Read the model definition and answer for the solid it produces. Units are mm, in the model's axes. Face numbers are marked on the shaded views. A direction names the side the tool comes from. Give positions to 0.01 mm unless a question says otherwise; leave off trailing zeros. Loops run counter-clockwise (first coordinate to the right, second up) from the corner with the lowest first, then second, coordinate; pieces in that order, holes last. Notation, with made-up numbers: (-6.5, 78) - (48.5, 78) arc R26 ccw to (48.5, 116) - close; hole circle Ø9 at (21, 72.5). An arc over 180 degrees is marked (long way). Put each result on its own line as item: value. Start each with the question number.
1. For a pull along X with two mould halves and no side action, classify the marked faces 1, 2 and 3 as released by +X, released by -X, zero draft, split by the parting line, or undercut.
2. Consider L1, parallel to Z at x = -20, y = 6; L2, parallel to Y at x = -5, z = -15; L3, parallel to Y at x = 2, z = 20. Determine where each line is inside the solid, lowest interval first. Write a range as from..to.
3. A cutting plane is placed at C-C, the plane z = 2. Determine the outline of the cut face in (x, y).
4. A cutting plane is placed at B-B, the plane x = -16.5. Determine the outline of the cut face in (y, z).
5. A cutting plane is placed at D-D, the plane x = -58. Determine the outline of the cut face in (y, z), plus the area to 3 significant figures.
6. For the marked faces 4, 5 and 6, determine the directions among +Z, -Z, +X, -X, +Y, -Y from which every point of the face is accessible in a straight line to the end or side of a thin tool.
7. A cutting plane is placed at A-A, the plane y = 9. Determine the outline of the cut face in (x, z).
8. Given pin 1 Ø24 at (y, z) = (40.5, -5.5) entering from -X; pin 2 Ø1.3 at (x, z) = (29.5, 28) entering from +Y; pin 3 Ø11.5 at (x, z) = (-11.5, 31) entering from +Y, each flat-ended and moving along its own axis, determine where each tip first touches the part or whether it passes through.
```python
from build123d import *

# Parameters (mm, degrees)
SKETCH_W     = 60
SKETCH_H     = 85
PAD_DEPTH    = 1.2
SKETCH002_W  = 60
SKETCH002_H  = 1.2
PAD001_DEPTH = 80
SKETCH003_W  = 60
SKETCH003_H  = 1.2
PAD002_DEPTH = 60
SKETCH004_W  = 60
SKETCH004_H  = 1.2
PAD003_DEPTH = 35
SKETCH006_W  = 60
SKETCH006_H  = 2.4
PAD004_DEPTH = 4
SKETCH005_W  = 11.7
SKETCH005_H  = 2.4
PAD005_DEPTH = 18.6
SKETCH007_W  = 17
SKETCH007_H  = 0.8
PAD006_DEPTH = 36.6
SKETCH009_W  = 61.2
SKETCH009_H  = 1.2
PAD007_DEPTH = 35
SKETCH010_W  = 1.2
SKETCH010_H  = 60
PAD008_DEPTH = 78.8
SKETCH011_W  = 1.2
SKETCH011_H  = 22.6
PAD009_DEPTH = 32.6
FILLET_R     = 1
FILLET001_R  = 1
FILLET002_R  = 1
FILLET003_R  = 1
FILLET004_R  = 1
FILLET005_R  = 1
FILLET006_R  = 1
FILLET007_R  = 1
FILLET008_R  = 1
FILLET009_R  = 1
FILLET010_R  = 1
FILLET011_R  = 1
FILLET012_R  = 1
FILLET013_R  = 1
FILLET014_R  = 0.4
FILLET015_R  = 0.4
SKETCH012_W  = 16
SKETCH012_H  = 8
POCKET_DEPTH = 95.001


with BuildPart() as part:
    # Sketch → Pad (new body)
    with BuildSketch(Plane.XZ):
        Rectangle(SKETCH_W, SKETCH_H)
    extrude(amount=PAD_DEPTH)

    # Sketch002 (on Face5 of Pad) → Pad001 (join)
    with BuildSketch(Plane(origin=(0, 0, 0), x_dir=(1, 0, 0), z_dir=(0, 1, 0))):
        with Locations((0, 41.9)):
            Rectangle(SKETCH002_W, SKETCH002_H)
    extrude(amount=PAD001_DEPTH)

    # Sketch003 (on Face4 of Pad001) → Pad002 (join)
    with BuildSketch(Plane(origin=(0, 0, -41.3), x_dir=(-1, 0, 0), z_dir=(0, 0, 1))):
        with Locations((0, -79.4)):
            Rectangle(SKETCH003_W, SKETCH003_H)
    extrude(amount=PAD002_DEPTH)

    # Sketch004 (on Face2 of Pad002) → Pad003 (join)
    with BuildSketch(Plane(origin=(0, 0, 0), x_dir=(1, 0, 0), z_dir=(0, 1, 0))):
        with Locations((0, -41.9)):
            Rectangle(SKETCH004_W, SKETCH004_H)
    extrude(amount=PAD003_DEPTH)

    # Sketch006 (on Face7 of Pad003) → Pad004 (join)
    with BuildSketch(Plane(origin=(0, 0, 41.3), x_dir=(1, 0, 0), z_dir=(0, 0, -1))):
        with Locations((0, -33.8)):
            Rectangle(SKETCH006_W, SKETCH006_H)
    extrude(amount=PAD004_DEPTH)

    # Sketch005 (on Face11 of Pad004) → Pad005 (join)
    with BuildSketch(Plane(origin=(0, 0, 37.3), x_dir=(1, 0, 0), z_dir=(0, 0, -1))):
        with Locations((24.15, -33.8)):
            Rectangle(SKETCH005_W, SKETCH005_H)
        with Locations((-24.15, -33.8)):
            Rectangle(SKETCH005_W, SKETCH005_H)
    extrude(amount=PAD005_DEPTH)

    # Sketch007 (on Face12 of Pad005) → Pad006 (join)
    with BuildSketch(Plane(origin=(-18.3, 0, 0), x_dir=(0, 0, 1), z_dir=(1, 0, 0))):
        with Locations((28, -33.8)):
            Rectangle(SKETCH007_W, SKETCH007_H)
    extrude(amount=PAD006_DEPTH)

    # Sketch009 (on Face2 of Pad006) → Pad007 (join)
    with BuildSketch(Plane(origin=(-30, 0, 0), x_dir=(0, 0, -1), z_dir=(-1, 0, 0))):
        with Locations((11.9, -79.4)):
            Rectangle(SKETCH009_W, SKETCH009_H)
    extrude(amount=PAD007_DEPTH)

    # Sketch010 (on Face22 of Pad007) → Pad008 (join)
    with BuildSketch(Plane.XZ.offset(-78.8)):
        with Locations((29.4, -11.3)):
            Rectangle(SKETCH010_W, SKETCH010_H)
    extrude(amount=PAD008_DEPTH)

    # Sketch011 (on Face9 of Pad008) → Pad009 (join)
    with BuildSketch(Plane.XZ.offset(-32.6)):
        with Locations((29.4, 30)):
            Rectangle(SKETCH011_W, SKETCH011_H)
    extrude(amount=PAD009_DEPTH)

    # Fillet
    fillet_edges = [part.edges().sort_by_distance(p)[0] for p in [
        (0, 35, 42.5),
    ]]
    fillet(fillet_edges, radius=FILLET_R)

    # Fillet001
    fillet001_edges = [part.edges().sort_by_distance(p)[0] for p in [
        (0, -1.2, 42.5),
    ]]
    fillet(fillet001_edges, radius=FILLET001_R)

    # Fillet002
    fillet002_edges = [part.edges().sort_by_distance(p)[0] for p in [
        (-0.6, 0, 41.3),
    ]]
    fillet(fillet002_edges, radius=FILLET002_R)

    # Fillet003
    fillet003_edges = [part.edges().sort_by_distance(p)[0] for p in [
        (-0.6, 32.6, 41.3),
    ]]
    fillet(fillet003_edges, radius=FILLET003_R)

    # Fillet004
    fillet004_edges = [part.edges().sort_by_distance(p)[0] for p in [
        (-24.15, 32.6, 18.7),
    ]]
    fillet(fillet004_edges, radius=FILLET004_R)

    # Fillet005
    fillet005_edges = [part.edges().sort_by_distance(p)[0] for p in [
        (-24.15, 35, 18.7),
    ]]
    fillet(fillet005_edges, radius=FILLET005_R)

    # Fillet006
    fillet006_edges = [part.edges().sort_by_distance(p)[0] for p in [
        (23.55, 35, 18.7),
    ]]
    fillet(fillet006_edges, radius=FILLET006_R)

    # Fillet007
    fillet007_edges = [part.edges().sort_by_distance(p)[0] for p in [
        (23.55, 32.6, 18.7),
    ]]
    fillet(fillet007_edges, radius=FILLET007_R)

    # Fillet008
    fillet008_edges = [part.edges().sort_by_distance(p)[0] for p in [
        (0, 32.6, 37.3),
    ]]
    fillet(fillet008_edges, radius=FILLET008_R)

    # Fillet009
    fillet009_edges = [part.edges().sort_by_distance(p)[0] for p in [
        (0, 35, 37.3),
    ]]
    fillet(fillet009_edges, radius=FILLET009_R)

    # Fillet010
    fillet010_edges = [part.edges().sort_by_distance(p)[0] for p in [
        (0, -1.2, -42.5),
    ]]
    fillet(fillet010_edges, radius=FILLET010_R)

    # Fillet011
    fillet011_edges = [part.edges().sort_by_distance(p)[0] for p in [
        (-17.5, 80, -42.5),
    ]]
    fillet(fillet011_edges, radius=FILLET011_R)

    # Fillet012
    fillet012_edges = [part.edges().sort_by_distance(p)[0] for p in [
        (-0.6, 78.8, -41.3),
    ]]
    fillet(fillet012_edges, radius=FILLET012_R)

    # Fillet013
    fillet013_edges = [part.edges().sort_by_distance(p)[0] for p in [
        (-0.6, 0, -41.3),
    ]]
    fillet(fillet013_edges, radius=FILLET013_R)

    # Fillet014
    fillet014_edges = [part.edges().sort_by_distance(p)[0] for p in [
        (-17.5, 80, 18.7),
    ]]
    fillet(fillet014_edges, radius=FILLET014_R)

    # Fillet015
    fillet015_edges = [part.edges().sort_by_distance(p)[0] for p in [
        (-18.1, 78.8, 18.7),
    ]]
    fillet(fillet015_edges, radius=FILLET015_R)

    # Sketch012 (on Face23 of Pad009) → Pocket (cut, through all)
    with BuildSketch(Plane(origin=(30, 0, 0), x_dir=(0, 0, 1), z_dir=(1, 0, 0))):
        with Locations((28.1, -10)):
            Rectangle(SKETCH012_W, SKETCH012_H)
    extrude(amount=-POCKET_DEPTH, mode=Mode.SUBTRACT)


solid = part.part
```
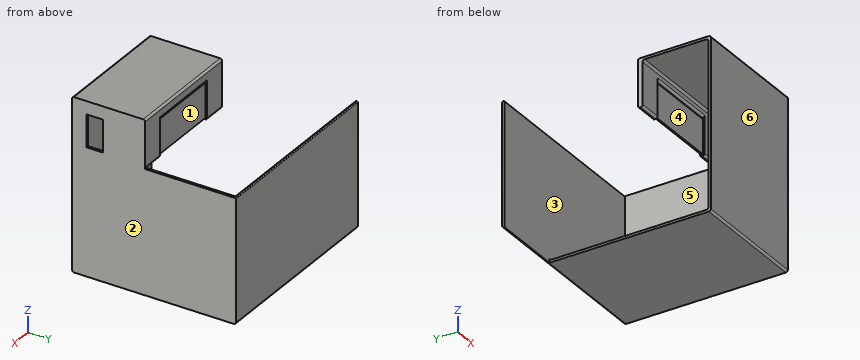
Return value:
1. face 1: undercut
1. face 2: released by +X
1. face 3: zero draft
2. L1: z = -42.5..-41.3, 41.3..42.5
2. L2: y = -1.2..0, 78.8..80
2. L3: y = -1.2..0, 33.4..34.2
3. outline: (-65, 78.8) - (28.8, 78.8) - (28.8, 0) - (-30, 0) - (-30, -1.2) - (30, -1.2) - (30, 80) - (-65, 80) - close
4. outline: (-1.2, -41.5) arc R1 ccw to (-0.2, -42.5) - (79, -42.5) arc R1 ccw to (80, -41.5) - (80, 18.3) arc R0.4 ccw to (79.6, 18.7) - (79.2, 18.7) arc R0.4 ccw to (78.8, 18.3) - (78.8, -40.3) arc R1 cw to (77.8, -41.3) - (1, -41.3) arc R1 cw to (0, -40.3) - (0, 40.3) arc R1 cw to (1, 41.3) - (31.6, 41.3) arc R1 cw to (32.6, 40.3) - (32.6, 38.3) arc R1 ccw to (33.6, 37.3) - (34, 37.3) arc R1 ccw to (35, 38.3) - (35, 41.5) arc R1 ccw to (34, 42.5) - (-0.2, 42.5) arc R1 ccw to (-1.2, 41.5) - close; (33.4, 19.5) - (34.2, 19.5) - (34.2, 36.5) - (33.4, 36.5) - close
5. outline: (78.8, -42.5) - (79, -42.5) arc R1 ccw to (80, -41.5) - (80, 18.3) arc R0.4 ccw to (79.6, 18.7) - (79.2, 18.7) arc R0.4 ccw to (78.8, 18.3) - close
5. area: 73.2 mm2
6. face 4: none
6. face 5: -X
6. face 6: +Z, -Z, +X, -X, -Y
7. outline: (-30, -42.5) - (30, -42.5) - (30, 20.1) - (28.8, 20.1) - (28.8, -41.3) - (-30, -41.3) - close; (-30, 41.3) - (28.8, 41.3) - (28.8, 36.1) - (30, 36.1) - (30, 42.5) - (-30, 42.5) - close
8. pin 1: stops at x = 28.8
8. pin 2: stops at y = 35
8. pin 3: stops at y = 34.2
